Source: CAD feature listing. Evaluate the final solid. Frame: model axes, mm. A direction names the side the tool comes from. Give positions to 0.01 mm unless a question says otherwise; leave off trailing zeros. Order: outer loops, then holes, each group sorted by start corner. A loop starts at its lowest first (then second) coordinate and runs counter-clockwise, first axis right, second up. Notation, with made-up numbers: M 80.25,-16 L 91.25,-16 A19 ccw 91.25,2 Z; hole C 8.25,-1 d5. An arc over 180 degrees is marked long. Use CSV: the item, a comma, the result in double quotes. Start each with the question number.
Item 1: Access query for faces 4 (the face through (23.8, 7.6, 9)), 5 (the face through (62.2, 7.6, 9)), 6 (the face through (-6, 20, 6)), 7 (the face through (81, 17.5, 6)). Directions: +Z, -Z, +X, -X, +Y, -Y. A direction counts if a zero-diameter tool reaches every point of the face in a straight line with its end or side. Return the directions, or none.
Item 2: Section query A-A on y = 7.5. Return loops of the section in (x, z).
Item 3: Pull-direction query (X, two-part tool) for faces 1 (the face through (21.685, 10.879, 6.084)), 2 (the face through (42, 0, 6)), 3 (the face through (25, 53, 6)); classes: +X half, -X half, draft (parallel to the pull), parting line (faces both ways), or undercut.
Item 4: Section query B-B on x = 68. Return loops of the section in (y, z), and give its area (3 significant figures).
Item 5: Section query D-D on y = 29.5. Return loops of the section in (x, z).
Item 6: Section query C-C on z = 1.75. Return loops of the section in (x, y).
Item 7: Ray query, probe 1 along Y at (x, z) = (18, 8.75); probe 2 along Y at (x, z) = (77, 6); probe 3 along Y at (x, z) = (72, 8.25). Return the intervals inside material, ascending. Write a range as from..to.
Item 8: First-contact query: pin 1 (3.5 mm diameter, centred on y = 9.5, z = 7.5, fed in from -X); pin 2 (6 mm diameter, centred on y = 27, z = 7, fed in from +X); pin 3 (3.5 mm diameter, centred on y = 52.5, z = 6, fed in from -X). Flat tips, straight axial feed; report the tip coordinate or a pass-through.
from build123d import *

# Parameters (mm, degrees)
SKETCH1_W           = 86
SKETCH1_H           = 60
BOSS_EXTRUDE1_DEPTH = 12
CUT_EXTRUDE1_REACH  = 107.546
SKETCH2_W           = 20
SKETCH2_H           = 25
SKETCH3_W           = 24
SKETCH3_H           = 20
BOSS_EXTRUDE2_DEPTH = 12
CUT_EXTRUDE2_REACH  = 107.546
SKETCH4_R           = 5
SKETCH5_R           = 3
CUT_EXTRUDE3_DEPTH  = 25


with BuildPart() as part:
    # Sketch1 → Boss-Extrude1 (new body)
    with BuildSketch(Plane.XY):
        with Locations((43, 30)):
            Rectangle(SKETCH1_W, SKETCH1_H)
    extrude(amount=BOSS_EXTRUDE1_DEPTH)

    # Sketch2 → Cut-Extrude1 (cut, up to next)
    with BuildSketch(Plane.XY.offset(12), mode=Mode.PRIVATE) as cut_extrude1_sk1:
        with Locations((86, 30)):
            Rectangle(SKETCH2_W, SKETCH2_H)
    cut_extrude1_tool1 = extrude(cut_extrude1_sk1.sketch, amount=-CUT_EXTRUDE1_REACH, mode=Mode.PRIVATE) & part.part
    add(cut_extrude1_tool1.solids().sort_by_distance((86, 30, 12))[0], mode=Mode.SUBTRACT)

    # Sketch3 → Boss-Extrude2 (add)
    with BuildSketch(Plane.XY.offset(12)):
        with Locations((0, 30)):
            Rectangle(SKETCH3_W, SKETCH3_H)
    extrude(amount=-BOSS_EXTRUDE2_DEPTH)

    # Sketch4 → Cut-Extrude2 (cut, up to next)
    with BuildSketch(Plane.XY.offset(12), mode=Mode.PRIVATE) as cut_extrude2_sk1:
        with Locations((68, 52.5)):
            Circle(SKETCH4_R)
    cut_extrude2_tool1 = extrude(cut_extrude2_sk1.sketch, amount=-CUT_EXTRUDE2_REACH, mode=Mode.PRIVATE) & part.part
    # Sketch4 → Cut-Extrude2 (cut, up to next)
    with BuildSketch(Plane.XY.offset(12), mode=Mode.PRIVATE) as cut_extrude2_sk2:
        with Locations((68, 7.5)):
            Circle(SKETCH4_R)
    cut_extrude2_tool2 = extrude(cut_extrude2_sk2.sketch, amount=-CUT_EXTRUDE2_REACH, mode=Mode.PRIVATE) & part.part
    cut_extrude2_1 = cut_extrude2_tool1.solids().sort_by_distance((68, 52.5, 12))[0]
    add(cut_extrude2_1, mode=Mode.SUBTRACT)
    cut_extrude2_2 = cut_extrude2_tool2.solids().sort_by_distance((68, 7.5, 12))[0]
    add(cut_extrude2_2, mode=Mode.SUBTRACT)
    cut_extrude2 = cut_extrude2_1 + cut_extrude2_2  # Cut-Extrude2 as one shape, for the pattern or mirror that repeats it

    # Sketch5 → Cut-Extrude3 (cut)
    with BuildSketch(Plane(origin=(86, 0, 0), x_dir=(0, 0, -1), z_dir=(1, 0, 0))):
        with Locations((-6, 52.5)):
            Circle(SKETCH5_R)
        with Locations((-6, 7.5)):
            Circle(SKETCH5_R)
    cut_extrude3 = extrude(amount=-CUT_EXTRUDE3_DEPTH, mode=Mode.SUBTRACT)

    # Mirror2: Cut-Extrude2, Cut-Extrude3 across plane
    add(cut_extrude2.mirror(Plane.ZY.offset(-43)), mode=Mode.SUBTRACT)
    add(cut_extrude3.mirror(Plane.ZY.offset(-43)), mode=Mode.SUBTRACT)


solid = part.part
Verdict:
1,face 4,"-X"
1,face 5,"+X"
1,face 6,"+Z, -Z, -X, -Y"
1,face 7,"+Z, -Z, +X"
2,outline,"M 0,0 L 13,0 L 13,3 L 0,3 Z; M 0,9 L 13,9 L 13,12 L 0,12 Z; M 23,0 L 63,0 L 63,3 L 61,3 L 61,9 L 63,9 L 63,12 L 23,12 L 23,9 L 25,9 L 25,3 L 23,3 Z; M 73,0 L 86,0 L 86,3 L 73,3 Z; M 73,9 L 86,9 L 86,12 L 73,12 Z"
3,face 1,"undercut"
3,face 2,"draft"
3,face 3,"-X half"
4,outline,"M 0,0 L 2.5,0 L 2.5,12 L 0,12 Z; M 12.5,0 L 47.5,0 L 47.5,12 L 12.5,12 Z; M 57.5,0 L 60,0 L 60,12 L 57.5,12 Z"
4,area,"480 mm2"
5,outline,"M -12,0 L 76,0 L 76,12 L -12,12 Z"
6,outline,"M -12,20 L 0,20 L 0,0 L 86,0 L 86,17.5 L 76,17.5 L 76,42.5 L 86,42.5 L 86,60 L 0,60 L 0,40 L -12,40 Z; hole C 18,7.5 d10; hole C 18,52.5 d10; hole C 68,7.5 d10; hole C 68,52.5 d10"
7,probe 1,"0..2.5, 12.5..47.5, 57.5..60"
7,probe 2,"0..4.5, 10.5..17.5, 42.5..49.5, 55.5..60"
7,probe 3,"0..4.5, 10.5..49.5, 55.5..60"
8,pin 1,"x = 0"
8,pin 2,"x = 76"
8,pin 3,"x = 25"
